from build123d import *

# Parameters (mm, degrees)
SKETCH1_W           = 16
SKETCH1_H           = 16
BOSS_EXTRUDE1_DEPTH = 1.6
SKETCH2_OUTSIDE_W   = 22.536
SKETCH2_OUTSIDE_H   = 22.536
CUT_EXTRUDE1_DEPTH  = 1.6


with BuildPart() as part:
    # Sketch1 → Boss-Extrude1 (new body)
    with BuildSketch(Plane(origin=(0, 0, 0), x_dir=(1, 0, 0), z_dir=(0, 1, 0))):
        Rectangle(SKETCH1_W, SKETCH1_H)
    extrude(amount=BOSS_EXTRUDE1_DEPTH)

    # Sketch2 outside → Cut-Extrude1 (cut)
    with BuildSketch(Plane(origin=(0, 1.6, 0), x_dir=(1, 0, 0), z_dir=(0, 1, 0))):
        Rectangle(SKETCH2_OUTSIDE_W, SKETCH2_OUTSIDE_H)
        with BuildLine():
            Line((6.0045, 6.15), (-5.9955, 6.15))
            ThreePointArc((-5.9955, 6.15), (-7.339002884, 5.593502884), (-7.8955, 4.25))
            Line((-7.8955, 4.25), (-7.8955, -1.75))
            ThreePointArc((-7.8955, -1.75), (-7.339002884, -3.093502884), (-5.9955, -3.65))
            Line((-5.9955, -3.65), (6.0045, -3.65))
            ThreePointArc((6.0045, -3.65), (7.348002884, -3.093502884), (7.9045, -1.75))
            Line((7.9045, -1.75), (7.9045, 4.25))
            ThreePointArc((7.9045, 4.25), (7.348002884, 5.593502884), (6.0045, 6.15))
        make_face(mode=Mode.SUBTRACT)
    extrude(amount=-CUT_EXTRUDE1_DEPTH, mode=Mode.SUBTRACT)


solid = part.part
Input: part model. Units: mm. Frame: model coordinates. Round coordinates to 2 decimals unless told otherwise and drop trailing zeros. Write each loop counter-clockwise with the first axis right and the second up, starting at its lowest first coordinate (ties: lowest second). Pieces come first, ordered by that corner, then holes.
1) Cut plane A-A (y = 0.65). Return the cut outline in (x, z), then the cut area to 3 significant figures.
2) Cut plane B-B (z = 2.75). Return the cut outline in (x, y).
3) Cut plane C-C (z = -5). Return the cut outline in (x, y).
4) Contact query for a flat-ended pin moving along its axis: P1, Ø4, axis at x = 0.5, z = -1, coming from the -Y side. Output: stop coordinate, or through.
5) Ray query, L1, parallel to X at y = 0.8, z = 2; L2, parallel to X at y = 1.5, z = 2.5; L3, parallel to Z at x = 7, y = 1. Return the intervals inside material, ascending.
Geometry says:
1. outline: (-7.9, -4.25) arc R1.9 ccw to (-6, -6.15) - (6, -6.15) arc R1.9 ccw to (7.9, -4.25) - (7.9, 1.75) arc R1.9 ccw to (6, 3.65) - (-6, 3.65) arc R1.9 ccw to (-7.9, 1.75) - close
1. area: 152 mm2
2. outline: (-7.61, 0) - (7.62, 0) - (7.62, 1.6) - (-7.61, 1.6) - close
3. outline: (-7.74, 0) - (7.75, 0) - (7.75, 1.6) - (-7.74, 1.6) - close
4. P1: stops at y = 0
5. L1: x = -7.88 to 7.89
5. L2: x = -7.74 to 7.75
5. L3: z = -5.87 to 3.37
